The model under review builds one solid part; all positions refer to its coordinate system, in mm. A direction names the side the tool comes from. Coordinates: 2 decimals unless noted, no trailing zeros. Order: outer loops, then holes, each group sorted by start corner. A loop starts at its lowest first (then second) coordinate and runs counter-clockwise, first axis right, second up. Notation, with made-up numbers: M 87.25,26 L 143.25,26 A12 cw 143.25,31 Z; hole C 47.25,21 d8. An arc over 180 degrees is marked long. Answer as CSV lines item,"result". Start each with the question number.
Q1. Wall thickness on L1, parallel to Z at x = 15, y = 21; L2, parallel to Y at x = 16.2, z = 16; L3, parallel to X at y = 36, z = 5.5: over which ranges is each line inside the solid? List them lowest first. Write a range as [from, to].
Q2. Consider section B-B on z = 42. State how many separate pieces and enclosed holes the cut face has, and give its area (3 significant figures).
Q3. The part is to be moulded in two halves that separate along Z. For faces 1 (the face through (0, 44, 33)), 2 (the face through (-0.379, 4.93, -93.496)), 3 (the face through (-16, 14, -4.2)), 4 (the face through (-9, 36, 36.25)), say which applies: +Z half, -Z half, draft (parallel to the pull), parting line (faces both ways), or undercut.
Q4. Consider section D-D on y = 8. Write out the cut boundary in (x, z), and give its area (3 significant figures).
Q5. Machinability: for faces 5 (the face through (0, 27, -26.25)), 6 (the face through (16, 18.5, 2)), 7 (the face through (9, 36, 36.25)), which of the approach directions +Z, -Z, +X, -X, +Y, -Y give a long, thin tool a straight path to every point of the face, cutting with its end or side? Answer none if there is none.
Q6. For P1, Ø10, axis at x = -5, y = 24, coming from the -Z side; P2, Ø1.5, axis at x = 4.5, y = 5, coming from the -Z side; P3, Ø2, axis at x = 3, y = 6, coming from the -Z side, all flat-tipped, find the tip position at first contact; note any pin that passes through.
Q7. Consider section C-C on x = 0. Write out the cut boundary in (y, z).
Q8. Consider section A-A on z = 0.5. Write out the cut boundary in (x, y).
Autodesk Inventor part; units mm, degrees
ref_plane "YZ Plane" through (0, 0, 0) normal (1, 0, 0) x (0, 1, 0)
ref_plane "XZ Plane" through (0, 0, 0) normal (0, 1, 0) x (-1, 0, 0)
ref_plane "XY Plane" through (0, 0, 0) normal (0, 0, 1) x (1, 0, 0)
sketch "Sketch1" plane through (0, 0, 0) normal (0, 1, 0) x (-1, 0, 0)
  line L0 (-17.25, 26.25) -> (17.25, 26.25)
  line L1 (17.25, 26.25) -> (17.25, -26.25)
  line L2 (17.25, -26.25) -> (-17.25, -26.25)
  line L3 (-17.25, -26.25) -> (-17.25, 26.25)
  line L4 (-17.25, 26.25) -> (17.25, -26.25) construction
  line L5 (17.25, 26.25) -> (-17.25, -26.25) construction
  line L6 (17.25, -26.25) -> (-17.25, -26.25)
  line L7 (-17.25, -26.25) -> (-17.25, -76.25)
  line L8 (-17.25, -76.25) -> (17.25, -76.25)
  line L9 (17.25, -76.25) -> (17.25, -26.25)
  arc A0 (-17.25, -76.25) -> (17.25, -76.25) centre (0, -76.25) ccw
  point P0 (0, 0)
  dimension "d0" = 34.5
  dimension "d1" = 52.5
  dimension "d4" = 50
extrude "Floor" add sketch "Sketch1" along normal blind 10
sketch "Sketch3" plane through (0, 10, 0) normal (0, 1, 0) x (1, 0, 0)
  arc A0 (17.25, 76.25) -> (-17.25, 76.25) centre (0, 76.25) ccw
  circle A1 centre (0, 68.45) radius 10
  circle A2 centre (0, 68.45) radius 13
  line L0 (14.25, -23.25) -> (-14.25, -23.25)
  line L1 (-14.25, -23.25) -> (-14.25, 23.25)
  line L2 (-14.25, 23.25) -> (14.25, 23.25)
  line L3 (14.25, 23.25) -> (14.25, -23.25)
  line L4 (14.25, -23.25) -> (-14.25, 23.25) construction
  line L5 (-14.25, -23.25) -> (14.25, 23.25) construction
  line L6 (17.25, 26.25) -> (-17.25, 26.25)
  line L7 (-17.25, 26.25) -> (-17.25, -26.25)
  line L8 (-17.25, -26.25) -> (17.25, -26.25)
  line L9 (17.25, -26.25) -> (17.25, 26.25)
  line L10 (17.25, 26.25) -> (-17.25, -26.25) construction
  line L11 (-17.25, 26.25) -> (17.25, -26.25) construction
  line L12 (0, 23.25) -> (0, 68.45)
  point P0 (0, 0)
  dimension "d14" = 20
  dimension "d18" = 28.5
  dimension "d19" = 46.5
  dimension "d38" = 45.2
  dimension "d54" = 26
extrude "Slots" add sketch "Sketch3" along normal blind 34
sketch "Sketch4" plane through (17.25, 0, 26.25) normal (1, 0, 0) x (0, 0, -1)
  line L0 (3, 10) -> (49.5, 10)
  line L1 (49.5, 10) -> (49.5, 44)
  line L2 (49.5, 44) -> (3, 44)
  line L3 (3, 44) -> (3, 10)
  line L4 (26.25, 10) -> (38.25, 10)
  line L5 (3, 10) -> (49.5, 10)
  line L6 (38.25, 10) -> (14.25, 10)
  line L7 (10.25, 33) -> (34.25, 33)
  line L8 (34.25, 33) -> (34.25, 21)
  line L9 (34.25, 21) -> (10.25, 21)
  line L10 (10.25, 21) -> (10.25, 33)
  line L11 (10.25, 33) -> (34.25, 21) construction
  line L12 (34.25, 33) -> (10.25, 21) construction
  circle A0 centre (10.25, 33) radius 1.35
  circle A1 centre (34.25, 33) radius 1.35
  circle A2 centre (34.25, 21) radius 1.35
  circle A3 centre (10.25, 21) radius 1.35
  line L13 (49.5, 10) -> (49.5, 44)
  line L14 (49.5, 27) -> (34.25, 27)
  line L15 (34.25, 27) -> (22.25, 27)
  point P0 (26.25, 0)
  point P1 (22.25, 27)
  dimension "d0" = 34.5
  dimension "d24" = 12
  dimension "d25" = 24
  dimension "d26" = 2.7
  dimension "d27" = 2.7
  dimension "d28" = 2.7
  dimension "d29" = 2.7
  dimension "d56" = 15.25
  dimension "d57" = 12
extrude "Screws/Sides" cut sketch "Sketch4" against normal through all contours A1 L7 L8 | L8 L7 A1 | A2 L9 L8 | L8 L9 A2 | A0 L10 L7 | L7 L10 A0 | A3 L10 L9 | L9 L10 A3
sketch "Sketch5" plane through (0, 44, 0) normal (0, 1, 0) x (1, 0, 0)
  line L0 (14.25, -21.25) -> (-14.25, -21.25)
  line L1 (-14.25, -21.25) -> (-14.25, 21.25)
  line L2 (-14.25, 21.25) -> (14.25, 21.25)
  line L3 (14.25, 21.25) -> (14.25, -21.25)
  line L4 (14.25, -21.25) -> (-14.25, 21.25) construction
  line L5 (-14.25, -21.25) -> (14.25, 21.25) construction
  line L6 (12.25, 23.25) -> (-12.25, 23.25)
  line L7 (-12.25, 23.25) -> (-12.25, -23.25)
  line L8 (-12.25, -23.25) -> (12.25, -23.25)
  line L9 (12.25, -23.25) -> (12.25, 23.25)
  line L10 (12.25, 23.25) -> (-12.25, -23.25) construction
  line L11 (-12.25, 23.25) -> (12.25, -23.25) construction
  line L12 (-12.25, 21.25) -> (-14.25, 21.25)
  line L13 (12.25, 23.25) -> (12.25, 21.25)
  line L14 (12.25, -21.25) -> (14.25, -21.25)
  line L15 (12.25, -23.25) -> (12.25, -21.25)
  line L16 (-14.25, -21.25) -> (-14.25, -23.25)
  line L17 (-14.25, -23.25) -> (-12.25, -23.25)
  line L18 (-14.25, -21.25) -> (-12.25, -23.25)
  line L19 (-14.25, -23.25) -> (-14.25, -21.25)
  line L20 (-14.25, 21.25) -> (-12.25, 23.25)
  line L21 (-14.25, 23.25) -> (-14.25, 21.25)
  line L22 (-14.25, -23.25) -> (-14.25, 23.25)
  line L23 (12.25, 23.25) -> (14.25, 23.25)
  line L24 (14.25, 23.25) -> (14.25, 21.25)
  line L25 (12.25, 23.25) -> (14.25, 21.25)
  line L26 (14.25, 23.25) -> (12.25, 23.25)
  line L27 (14.25, -23.25) -> (12.25, -23.25)
  line L28 (14.25, -23.25) -> (-14.25, -23.25)
  line L29 (14.25, -21.25) -> (12.25, -23.25)
  line L30 (14.25, -23.25) -> (14.25, -21.25)
  line L31 (14.25, 23.25) -> (14.25, -23.25)
  line L32 (-14.25, 23.25) -> (-12.25, 23.25)
  line L33 (14.25, 23.25) -> (-14.25, 23.25)
  point P0 (0, 0)
  dimension "d32" = 42.5
  dimension "d33" = 24.5
extrude "Servo Corners" add sketch "Sketch5" against normal blind 34 contours L30 L27 L29 | L25 L23 L24 | L17 L16 L18 | L20 L21 L32
sketch "Sketch6" plane through (0, 44, 0) normal (0, 1, 0) x (1, 0, 0)
  line L0 (-12.25, 23.25) -> (12.25, 23.25)
  line L1 (0, 23.25) -> (0, 12)
  circle A0 centre (0, 68.45) radius 10
  line L2 (0, 12) -> (0, 68.45)
  point P0 (0, 0)
  dimension "d36" = 11.25
  dimension "d37" = 56.45
sketch "Sketch7" plane through (-17.25, 0, 26.25) normal (0, 0, 1) x (1, 0, 0)
  line L0 (0, 0) -> (34.5, 0)
  line L1 (34.5, 0) -> (34.5, 44)
  line L2 (34.5, 44) -> (0, 44)
  line L3 (0, 44) -> (0, 0)
  point P0 (17.25, 0)
extrude "Mount Extension" add sketch "Sketch7" along normal blind 30
sketch "Sketch8" plane through (-17.25, 0, 56.25) normal (0, 0, 1) x (1, 0, 0)
  line L0 (17.25, 0) -> (17.25, 10)
  line L1 (29.5, 44) -> (5, 44)
  line L2 (17.25, 27) -> (17.25, 35.5)
  line L3 (34.5, 10) -> (34.5, 44)
  line L4 (0, 10) -> (0, 44)
  line L5 (17.25, 35.5) -> (8.625, 35.5)
  circle A0 centre (8.625, 35.5) radius 2.6035
  line L6 (17.25, 10) -> (8.625, 10)
  line L7 (29.5, 10) -> (5, 10)
  line L8 (8.625, 10) -> (8.625, 18.5)
  circle A1 centre (8.625, 18.5) radius 2.6035
  line L9 (34.5, 35.5) -> (25.875, 35.5)
  dimension "d41" = 10
  dimension "d42" = 5.207
  dimension "d43" = 8.5
  dimension "d44" = 5.207
  dimension "d47" = 8.625
extrude "Mount Holes" cut sketch "Sketch8" against normal blind 20
pattern_linear "Rectangular Pattern1" count 2 spacing 17.25 along (1, 0, 0) of "Mount Holes"
sketch "Sketch11" plane through (17.25, 0, -76.25) normal (1, 0, 0) x (0, 0, -1)
  line L0 (-85.05, 10) -> (-72.05, 10)
  line L1 (-72.05, 10) -> (-72.05, 18.5)
  line L2 (-72.05, 18.5) -> (-85.05, 18.5)
  line L3 (-85.05, 18.5) -> (-85.05, 10)
  circle A0 centre (-68.25, 21) radius 1.35
  line L4 (-68.25, 21) -> (-68.25, 10)
  line L5 (-97.5, 10) -> (-55, 10)
  line L6 (-68.25, 10) -> (-72.05, 10)
  point P0 (-76.25, 0)
  dimension "d58" = 13
  dimension "d59" = 8.5
  dimension "d60" = 3.8
extrude "Wiring Holes" cut sketch "Sketch11" against normal through all contours L3 L2 L1 L0
properties part number "JointBase"
Evaluation:
1,L1,"z = [-26.25, -9.35], [-6.65, 14.65], [17.35, 56.25]"
1,L2,"y = [0, 19.65], [22.35, 31.65], [34.35, 44]"
1,L3,"x = [-17.25, -14.25], [14.25, 17.25]"
2,separate pieces,"1"
2,enclosed holes,"4"
2,area,"1,430 mm²"
3,face 1,"draft"
3,face 2,"-Z half"
3,face 3,"undercut"
3,face 4,"+Z half"
4,outline,"M -17.25,-76.25 A17.25 ccw 17.25,-76.25 L 17.25,56.25 L -17.25,56.25 Z"
4,area,"5,040 mm²"
5,face 5,"+X, -X, +Y"
5,face 6,"+X, -X"
5,face 7,"+Z"
6,P1,"stops at z = -81.45"
6,P2,"stops at z = -93.09"
6,P3,"stops at z = -93.38"
7,outline,"M 0,-93.5 L 10,-93.5 L 10,-81.45 L 44,-81.45 L 44,-78.45 L 10,-78.45 L 10,-58.45 L 44,-58.45 L 44,-55.45 L 10,-55.45 L 10,-26.25 L 44,-26.25 L 44,-23.25 L 10,-23.25 L 10,23.25 L 44,23.25 L 44,56.25 L 0,56.25 Z"
8,outline,"M -17.25,0 L 17.25,0 L 17.25,10 L -17.25,10 Z; M -17.25,18.5 L -14.25,18.5 L -14.25,44 L -17.25,44 Z; M 14.25,18.5 L 17.25,18.5 L 17.25,44 L 14.25,44 Z"
